Geometry check sheet. Reference: the model listing, model coordinates, mm. Face numbers are marked on the shaded views. A direction names the side the tool comes from. Round coordinates to 2 decimals unless told otherwise and drop trailing zeros. Write each loop counter-clockwise with the first axis right and the second up, starting at its lowest first coordinate (ties: lowest second). Pieces come first, ordered by that corner, then holes.
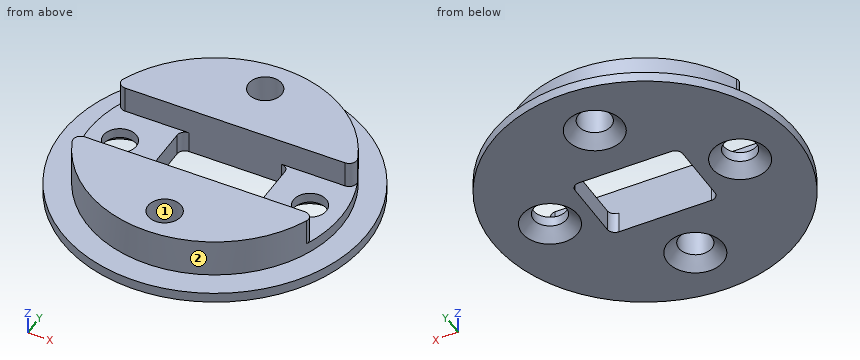
from build123d import *

# Parameters (mm, degrees)
SKIZZE14_W                                           = 8.5
SKIZZE14_H                                           = 6
SCHNITT_LINEAR_AUSTRAGEN4_DEPTH                      = 4.8
SKIZZE15_W                                           = 24
SKIZZE15_H                                           = 6
SCHNITT_LINEAR_AUSTRAGEN5_DEPTH                      = 2.1
VERRUNDUNG1_R                                        = 0.6
VERRUNDUNG2_R                                        = 0.6
FORMSENKUNG_F_R_M2_LINSENSENKSCHRAUBE_MI_D           = 2.6
FORMSENKUNG_F_R_M2_LINSENSENKSCHRAUBE_MI_CSINK_D     = 4.4
FORMSENKUNG_F_R_M2_LINSENSENKSCHRAUBE_MI_CSINK_ANGLE = 90
FORMSENKUNG_F_R_M2_LINSENSENKSCHRAUB_2_D             = 2.6
FORMSENKUNG_F_R_M2_LINSENSENKSCHRAUB_2_CSINK_D       = 4.4
FORMSENKUNG_F_R_M2_LINSENSENKSCHRAUB_2_CSINK_ANGLE   = 90


with BuildPart() as part:
    # Skizze2 → Rotation1 (revolve)
    with BuildSketch(Plane(origin=(0, 0, 0), x_dir=(1, 0, 0), z_dir=(0, 1, 0))):
        Polygon((0, 0), (10, 0), (10, 3), (12, 3), (12, 3.8), (0, 3.8), align=None)
    revolve(axis=Axis((0, 0, -3.8), (0, 0, 1)))

    # Skizze14 → Schnitt-Linear austragen4 (cut, through all)
    with BuildSketch(Plane.XY):
        Rectangle(SKIZZE14_W, SKIZZE14_H)
    extrude(amount=-SCHNITT_LINEAR_AUSTRAGEN4_DEPTH, mode=Mode.SUBTRACT)

    # Skizze15 → Schnitt-Linear austragen5 (cut)
    with BuildSketch(Plane.XY):
        Rectangle(SKIZZE15_W, SKIZZE15_H)
    extrude(amount=-SCHNITT_LINEAR_AUSTRAGEN5_DEPTH, mode=Mode.SUBTRACT)

    # Verrundung1
    verrundung1_edges = [part.edges().sort_by_distance(p)[0] for p in [
        (4.25, 3, -2.95),
        (4.25, -3, -2.95),
        (-4.25, -3, -2.95),
        (-4.25, 3, -2.95),
    ]]
    fillet(verrundung1_edges, radius=VERRUNDUNG1_R)

    # Verrundung2
    verrundung2_edges = [part.edges().sort_by_distance(p)[0] for p in [
        (-9.539392014, -3, -1.05),
        (9.539392014, -3, -1.05),
        (9.539392014, 3, -1.05),
        (-9.539392014, 3, -1.05),
    ]]
    fillet(verrundung2_edges, radius=VERRUNDUNG2_R)

    # Formsenkung f_r M2 Linsensenkschraube mi (through all)
    with Locations(Plane(origin=(0, 0, -3.8), x_dir=(1, 0, 0), z_dir=(0, 0, -1))):
        with Locations((-7.5, 0), (7.5, 0)):
            CounterSinkHole(FORMSENKUNG_F_R_M2_LINSENSENKSCHRAUBE_MI_D / 2, FORMSENKUNG_F_R_M2_LINSENSENKSCHRAUBE_MI_CSINK_D / 2, counter_sink_angle=FORMSENKUNG_F_R_M2_LINSENSENKSCHRAUBE_MI_CSINK_ANGLE)

    # Formsenkung f_r M2 Linsensenkschraub 2 (through all)
    with Locations(Plane(origin=(0, 0, -3.8), x_dir=(-1, 0, 0), z_dir=(0, 0, -1))):
        with Locations((0, 7.5), (0, -7.5)):
            CounterSinkHole(FORMSENKUNG_F_R_M2_LINSENSENKSCHRAUB_2_D / 2, FORMSENKUNG_F_R_M2_LINSENSENKSCHRAUB_2_CSINK_D / 2, counter_sink_angle=FORMSENKUNG_F_R_M2_LINSENSENKSCHRAUB_2_CSINK_ANGLE)


solid = part.part
1. Scan lines: line 1 along Y through (x, z) = (0, -1.5); line 2 along X through (y, z) = (-7.5, -1.45); line 3 along Y through (x, z) = (3, -3.45). Record each from-to range of solid material in increasing order.
2. Access from +Z, -Z, +X, -X, +Y, -Y to the whole of each face (thin tool, end or side, straight path). Record for the marked faces 1 and 2.
3. Section check A-A (y = 0). Record the cut outline in (x, z).
4. Section check B-B (z = -0.75). Record the cut outline in (x, y).
5. Depth check by flat-ended pin: pin 1 Ø2 at (x, y) = (0, -7.5) entering from -Z; pin 2 Ø1 at (x, z) = (3, -1) entering from -Y; pin 3 Ø1.9 at (x, y) = (-7.5, 1.5) entering from +Z; pin 4 Ø2 at (x, z) = (-7, -0.5) entering from +Y. Enter the tip coordinate at first touch or a pass-through.
6. Section check D-D (y = -7.5). Record the cut outline in (x, z), plus the area to 3 significant figures.
7. Section check C-C (x = 0). Record the cut outline in (y, z), plus the area to 3 significant figures.
Results below:
1. line 1: y = -10 to -8.8, -6.2 to -3, 3 to 6.2, 8.8 to 10
1. line 2: x = -6.61 to -1.3, 1.3 to 6.61
1. line 3: y = -11.62 to -3, 3 to 11.62
2. face 1: +Z, -Z
2. face 2: +Z
3. outline: (-12, -3.8) - (-9.7, -3.8) - (-8.8, -2.9) - (-8.8, -2.1) - (-10, -2.1) - (-10, -3) - (-12, -3) - close; (-6.2, -2.9) - (-5.3, -3.8) - (-4.25, -3.8) - (-4.25, -2.1) - (-6.2, -2.1) - close; (4.25, -3.8) - (5.3, -3.8) - (6.2, -2.9) - (6.2, -2.1) - (4.25, -2.1) - close; (8.8, -2.9) - (9.7, -3.8) - (12, -3.8) - (12, -3) - (10, -3) - (10, -2.1) - (8.8, -2.1) - close
4. outline: (-9.24, -3.83) arc R10 ccw to (9.24, -3.83) arc R0.6 ccw to (8.68, -3) - (-8.68, -3) arc R0.6 ccw to start; (-9.24, 3.83) arc R0.6 ccw to (-8.68, 3) - (8.68, 3) arc R0.6 ccw to (9.24, 3.83) arc R10 ccw to start; hole circle Ø2.6 at (0, -7.5); hole circle Ø2.6 at (0, 7.5)
5. pin 1: passes through
5. pin 2: stops at y = -9.68
5. pin 3: stops at z = -2.1
5. pin 4: stops at y = 8
6. outline: (-9.37, -3.8) - (-2.2, -3.8) - (-1.3, -2.9) - (-1.3, 0) - (-6.61, 0) - (-6.61, -3) - (-9.37, -3) - close; (1.3, -2.9) - (2.2, -3.8) - (9.37, -3.8) - (9.37, -3) - (6.61, -3) - (6.61, 0) - (1.3, 0) - close
6. area: 44.0 mm2
7. outline: (-12, -3.8) - (-9.7, -3.8) - (-8.8, -2.9) - (-8.8, 0) - (-10, 0) - (-10, -3) - (-12, -3) - close; (-6.2, -2.9) - (-5.3, -3.8) - (-3, -3.8) - (-3, 0) - (-6.2, 0) - close; (3, -3.8) - (5.3, -3.8) - (6.2, -2.9) - (6.2, 0) - (3, 0) - close; (8.8, -2.9) - (9.7, -3.8) - (12, -3.8) - (12, -3) - (10, -3) - (10, 0) - (8.8, 0) - close
7. area: 35.0 mm2
